from build123d import *

# Parameters (mm, degrees)
SKETCH1_W           = 230
SKETCH1_H           = 150
BOSS_EXTRUDE1_DEPTH = 5
CUT_EXTRUDE1_DEPTH  = 275.636122897


with BuildPart() as part:
    # Sketch1 → Boss-Extrude1 (new body)
    with BuildSketch(Plane(origin=(0, 0, 0), x_dir=(1, 0, 0), z_dir=(0, 1, 0))):
        with Locations((115, -75)):
            Rectangle(SKETCH1_W, SKETCH1_H)
    extrude(amount=BOSS_EXTRUDE1_DEPTH)

    # Sketch2 → Cut-Extrude1 (cut, through all)
    with BuildSketch(Plane(origin=(0, 5, 0), x_dir=(1, 0, 0), z_dir=(0, 1, 0))):
        Polygon((145, 0), (85, 0), (85, -40), (115, -57.320508076), (145, -40), align=None)
    extrude(amount=-CUT_EXTRUDE1_DEPTH, mode=Mode.SUBTRACT)


solid = part.part
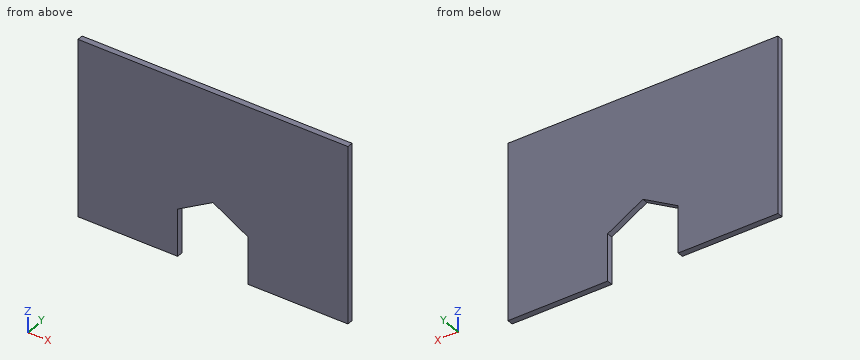
Build history of the part. All positions in model axes, mm. Round coordinates to 2 decimals unless told otherwise and drop trailing zeros. Loops run counter-clockwise (first coordinate to the right, second up) from the corner with the lowest first, then second, coordinate; pieces in that order, holes last. Notation, with made-up numbers: (12.25, 6) -> (60.25, 6) arc R34 cw to (60.25, 45) -> close; hole circle Ø2 at (66.5, -23). An arc over 180 degrees is marked (long way). One line per item, written item: value. Start each with the question number.
Q1. Cut at C-C on z = 48.5. List the corners of the cut face in (x, y).
Q2. Probe line 1 along X through (y, z) = (1.25, 36.5); line 2 along X through (y, z) = (2.55, 55); line 3 along Z through (x, y) = (122.5, 2.2). List the from-to ranges inside material, lowest first.
Q3. Cut at D-D on x = 141.5. List the corners of the cut face in (y, z), plus the area to 3 significant figures.
Q4. Drop a flat-ended pin along its axis: pin 1 Ø1.5 at (y, z) = (1, 94) entering from -X. Give the stop position or say it passes through.
Q5. Cut at A-A on z = 15.5. List the corners of the cut face in (x, y), plus the area to 3 significant figures.
Q6. Cut at B-B on y = 1.9. List the corners of the cut face in (x, z).
Computed:
1. outline: (0, 0) -> (99.72, 0) -> (99.72, 5) -> (0, 5) -> close; (130.28, 0) -> (230, 0) -> (230, 5) -> (130.28, 5) -> close
2. line 1: 0 to 85, 145 to 230
2. line 2: 0 to 110.98, 119.02 to 230
2. line 3: 52.99 to 150
3. outline: (0, 42.02) -> (5, 42.02) -> (5, 150) -> (0, 150) -> close
3. area: 540 mm²
4. pin 1: x = 0
5. outline: (0, 0) -> (85, 0) -> (85, 5) -> (0, 5) -> close; (145, 0) -> (230, 0) -> (230, 5) -> (145, 5) -> close
5. area: 850 mm²
6. outline: (0, 0) -> (85, 0) -> (85, 40) -> (115, 57.32) -> (145, 40) -> (145, 0) -> (230, 0) -> (230, 150) -> (0, 150) -> close
